```python
from build123d import *

# Parameters (mm, degrees)
SKETCH_1_W          = 42.110617321
SKETCH_1_H          = 5
EXTRUDE_1_DEPTH     = 5
SKETCH_2_W          = 13
SKETCH_2_H          = 5
EXTRUDE_2_DEPTH     = 25
SKETCH_2_3_W        = 5
SKETCH_2_3_H        = 5
EXTRUDE_3_DEPTH     = 15
SKETCH_3_W          = 5
SKETCH_3_H          = 15
EXTRUDE_4_DEPTH     = 7
SKETCH_4_R          = 2
CUT_EXTRUDE_1_DEPTH = 61.919456182
SKETCH_4_3_R        = 3.1
CUT_EXTRUDE_2_DEPTH = 2.7


with BuildPart() as part:
    # Sketch 1 → Extrude 1 (new body)
    with BuildSketch(Plane(origin=(0, 0, 0), x_dir=(1, 0, 0), z_dir=(0, 1, 0))):
        with Locations((-21.05530866, 2.5)):
            Rectangle(SKETCH_1_W, SKETCH_1_H)
    extrude(amount=EXTRUDE_1_DEPTH)

    # Sketch 2 → Extrude 2 (add)
    with BuildSketch(Plane(origin=(0, 0, 0), x_dir=(-1, 0, 0), z_dir=(0, 0, -1))):
        with Locations((-6.5, 2.5)):
            Rectangle(SKETCH_2_W, SKETCH_2_H)
    extrude(amount=EXTRUDE_2_DEPTH)

    # Sketch 2_3 → Extrude 3 (add)
    with BuildSketch(Plane(origin=(0, 0, 0), x_dir=(-1, 0, 0), z_dir=(0, 0, -1))):
        with Locations((-10.5, 2.5)):
            Rectangle(SKETCH_2_3_W, SKETCH_2_3_H)
    extrude(amount=-EXTRUDE_3_DEPTH)

    # Sketch 3 → Extrude 4 (add)
    with BuildSketch(Plane.XZ):
        Polygon((8, 0), (-42.110617321, 0), (-42.110617321, -5), (13, -5), (13, 0), align=None)
        with Locations((10.5, 7.5)):
            Rectangle(SKETCH_3_W, SKETCH_3_H)
    extrude(amount=EXTRUDE_4_DEPTH)

    # Sketch 4 → Cut-Extrude 1 (cut, through all)
    with BuildSketch(Plane(origin=(13, 0, 0), x_dir=(0, 0, -1), z_dir=(1, 0, 0))):
        with Locations(Location((-9, -1, 0), (0, 0, 90))):
            Circle(SKETCH_4_R)
    extrude(amount=-CUT_EXTRUDE_1_DEPTH, mode=Mode.SUBTRACT)

    # Sketch 4_3 → Cut-Extrude 2 (cut)
    with BuildSketch(Plane(origin=(13, 0, 0), x_dir=(0, 0, -1), z_dir=(1, 0, 0))):
        with Locations(Location((-9, -1, 0), (0, 0, 90))):
            Circle(SKETCH_4_3_R)
    extrude(amount=-CUT_EXTRUDE_2_DEPTH, mode=Mode.SUBTRACT)


solid = part.part
```
Work out the finished part from the listing and answer in its coordinate system (mm). A direction names the side the tool comes from. Round coordinates to 2 decimals unless told otherwise and drop trailing zeros. Write each loop counter-clockwise with the first axis right and the second up, starting at its lowest first coordinate (ties: lowest second). Pieces come first, ordered by that corner, then holes.
1) Flat-ended cylindrical pins translate along their axes: P1, Ø4, axis at y = -5, z = 8.5, coming from the -X side; P2, Ø5, axis at y = -1, z = 9, coming from the +X side; P3, Ø6.5, axis at x = 5.5, z = -14, coming from the -Y side; P4, Ø1.9, axis at y = 0, z = 9, coming from the +X side. Find the tip coordinate at first contact, or state that the pin passes through.
2) Which of the six approach directions +Z, -Z, +X, -X, +Y, -Y give full straight-line access (tool end or side, diameter ignored) to faces 1 (the face through (0, 2, -15)), 2 (the face through (11.67, 0.67, 11.61)), 3 (the face through (-17, -1, 0))?
3) A cutting plane is placed at C-C on x = 9.5. Determine the outline of the cut face in (y, z).
4) A cutting plane is placed at A-A on y = -1. Determine the outline of the cut face in (x, z), and give its area (3 significant figures).
5) Consider probe 1 along Z at (x, y) = (11.75, -1); probe 2 along Z at (x, y) = (9.6, -1); probe 3 along Z at (x, y) = (-17.5, -6). Determine where each line is inside the solid, lowest interval first.
6) A cutting plane is placed at B-B on z = 9. Determine the outline of the cut face in (x, y), and give its area (3 significant figures).
7) A cutting plane is placed at D-D on y = -5.5. Determine the outline of the cut face in (x, z), and give its area (3 significant figures).
8) Determine the mould class of faces 4 (the face through (7, 3, -25)), 5 (the face through (-2, 5, -4)), 6 (the face through (9, -1, 11)), 7 (the face through (10.3, 0, 7)) for opening direction Y: pulls with the +Y half, pulls with the -Y half, needs draft (parallel to the pull), parting line crosses it, or undercut.
Entries:
1. P1: stops at x = 8
1. P2: stops at x = 10.3
1. P3: stops at y = 0
1. P4: passes through
2. face 1: -Z, -X, +Y, -Y
2. face 2: +X
2. face 3: +Z, -X, +Y, -Y
3. outline: (-7, -5) - (0, -5) - (0, -25) - (5, -25) - (5, 15) - (-7, 15) - close; hole circle Ø4 at (-1, 9)
4. outline: (-42.11, -5) - (13, -5) - (13, 5.9) - (10.3, 5.9) - (10.3, 7) - (8, 7) - (8, 0) - (-42.11, 0) - close; (8, 11) - (10.3, 11) - (10.3, 12.1) - (13, 12.1) - (13, 15) - (8, 15) - close
4. area: 325 mm2
5. probe 1: z = -5 to 5.9, 12.1 to 15
5. probe 2: z = -5 to 7, 11 to 15
5. probe 3: z = -5 to 0
6. outline: (8, -7) - (13, -7) - (13, -4.1) - (10.3, -4.1) - (10.3, -3) - (8, -3) - close; (8, 1) - (10.3, 1) - (10.3, 2.1) - (13, 2.1) - (13, 5) - (8, 5) - close
6. area: 34.1 mm2
7. outline: (-42.11, -5) - (13, -5) - (13, 15) - (8, 15) - (8, 0) - (-42.11, 0) - close
7. area: 351 mm2
8. face 4: needs draft
8. face 5: pulls with the +Y half
8. face 6: undercut
8. face 7: undercut
